Verification items for the finished model (mm, model axes). A direction names the side the tool comes from. Coordinates: 2 decimals unless noted, no trailing zeros. Loops run counter-clockwise (first coordinate to the right, second up) from the corner with the lowest first, then second, coordinate; pieces in that order, holes last. Notation, with made-up numbers: (62, 80) -> (71, 80) arc R16 ccw to (71, 89) -> close; hole circle Ø4 at (83.5, 55.5). An arc over 180 degrees is marked (long way). Write item = value, one per line.
```python
from build123d import *

# Parameters (mm, degrees)
MAINBODYS_R           = 2.5
MAIN_BODY_DEPTH       = 2
M3X0_5_TAPPED_HOLE1_D = 2.5
GROOVED_CUT_DEPTH     = 6.338539126
GC_START              = -2
GC_CP_DEPTH           = 4
PRESSFITBODYS_R       = 2
PRESSFITBODYS_R_2     = 1.25
PRESS_FIT_BODY_DEPTH  = 1


# Read off the part's stored shape, not the designer's step: GC CP
with BuildPart() as part:
    # MainBodyS → MAIN BODY (new, symmetric)
    with BuildSketch(Plane(origin=(0, 0, 0), x_dir=(1, 0, 0), z_dir=(0, 1, 0))):
        with Locations(Location((0, 0, 0), (0, 0, 270))):
            Circle(MAINBODYS_R)
    extrude(amount=MAIN_BODY_DEPTH, both=True)

    # M3x0.5 Tapped Hole1 (through all)
    with Locations(Plane(origin=(0, 2, 0), x_dir=(1, 0, 0), z_dir=(0, 1, 0))):
        with Locations((0, 0)):
            Hole(M3X0_5_TAPPED_HOLE1_D / 2)

    # GroovedCutS → GROOVED CUT (cut, through all)
    with BuildSketch(Plane(origin=(0, 2, 0), x_dir=(1, 0, 0), z_dir=(0, 1, 0))):
        with BuildLine():
            Line((0, 2.25), (0.382129822, 2.470622755))
            ThreePointArc((0.382129822, 2.470622755), (0, 2.5), (-0.382129822, 2.470622755))
            Line((-0.382129822, 2.470622755), (0, 2.25))
        make_face()
    extrude(amount=-GROOVED_CUT_DEPTH, mode=Mode.SUBTRACT)

    # GC CP outline → GC CP (cut)
    with BuildSketch(Plane(origin=(0, 0, 0), x_dir=(1, 0, 0), z_dir=(0, 1, 0)).offset(GC_START)):
        with BuildLine():
            ThreePointArc((-0.727675966, 2.391754103), (-1.084709348, 2.25242217), (-1.416250112, 2.060154271))
            Line((-1.416250112, 2.060154271), (-0.976238413, 2.027179953))
            Line((-0.976238413, 2.027179953), (-0.727675966, 2.391754103))
        make_face()
        with BuildLine():
            Line((0.976238413, 2.027179953), (1.416250112, 2.060154271))
            ThreePointArc((1.416250112, 2.060154271), (1.084709348, 2.25242217), (0.727675966, 2.391754103))
            Line((0.727675966, 2.391754103), (0.976238413, 2.027179953))
        make_face()
        with BuildLine():
            Line((1.759120836, 1.402852054), (2.169864698, 1.241646967))
            ThreePointArc((2.169864698, 1.241646967), (1.954578706, 1.558724504), (1.693356605, 1.839169217))
            Line((1.693356605, 1.839169217), (1.759120836, 1.402852054))
        make_face()
        with BuildLine():
            Line((2.193587802, 0.500672101), (2.493710969, 0.177216254))
            ThreePointArc((2.493710969, 0.177216254), (2.43731978, 0.556302335), (2.3236472, 0.922314312))
            Line((2.3236472, 0.922314312), (2.193587802, 0.500672101))
        make_face()
        with BuildLine():
            Line((2.193587802, -0.500672101), (2.3236472, -0.922314312))
            ThreePointArc((2.3236472, -0.922314312), (2.43731978, -0.556302335), (2.493710969, -0.177216254))
            Line((2.493710969, -0.177216254), (2.193587802, -0.500672101))
        make_face()
        with BuildLine():
            Line((1.759120836, -1.402852054), (1.693356605, -1.839169217))
            ThreePointArc((1.693356605, -1.839169217), (1.954578706, -1.558724504), (2.169864698, -1.241646967))
            Line((2.169864698, -1.241646967), (1.759120836, -1.402852054))
        make_face()
        with BuildLine():
            Line((0.976238413, -2.027179953), (0.727675966, -2.391754103))
            ThreePointArc((0.727675966, -2.391754103), (1.084709348, -2.25242217), (1.416250112, -2.060154271))
            Line((1.416250112, -2.060154271), (0.976238413, -2.027179953))
        make_face()
        with BuildLine():
            Line((0, -2.25), (-0.382129822, -2.470622755))
            ThreePointArc((-0.382129822, -2.470622755), (0, -2.5), (0.382129822, -2.470622755))
            Line((0.382129822, -2.470622755), (0, -2.25))
        make_face()
        with BuildLine():
            Line((-0.976238413, -2.027179953), (-1.416250112, -2.060154271))
            ThreePointArc((-1.416250112, -2.060154271), (-1.084709348, -2.25242217), (-0.727675966, -2.391754103))
            Line((-0.727675966, -2.391754103), (-0.976238413, -2.027179953))
        make_face()
        with BuildLine():
            Line((-1.759120836, -1.402852054), (-2.169864698, -1.241646967))
            ThreePointArc((-2.169864698, -1.241646967), (-1.954578706, -1.558724504), (-1.693356605, -1.839169217))
            Line((-1.693356605, -1.839169217), (-1.759120836, -1.402852054))
        make_face()
        with BuildLine():
            Line((-2.193587802, -0.500672101), (-2.493710969, -0.177216254))
            ThreePointArc((-2.493710969, -0.177216254), (-2.43731978, -0.556302335), (-2.3236472, -0.922314312))
            Line((-2.3236472, -0.922314312), (-2.193587802, -0.500672101))
        make_face()
        with BuildLine():
            Line((-2.193587802, 0.500672101), (-2.3236472, 0.922314312))
            ThreePointArc((-2.3236472, 0.922314312), (-2.43731978, 0.556302335), (-2.493710969, 0.177216254))
            Line((-2.493710969, 0.177216254), (-2.193587802, 0.500672101))
        make_face()
        with BuildLine():
            Line((-1.759120836, 1.402852054), (-1.693356605, 1.839169217))
            ThreePointArc((-1.693356605, 1.839169217), (-1.954578706, 1.558724504), (-2.169864698, 1.241646967))
            Line((-2.169864698, 1.241646967), (-1.759120836, 1.402852054))
        make_face()
    extrude(amount=GC_CP_DEPTH, mode=Mode.SUBTRACT)

    # PressFitBodyS → PRESS FIT BODY (add)
    with BuildSketch(Plane(origin=(0, 2, 0), x_dir=(1, 0, 0), z_dir=(0, 1, 0))):
        with Locations(Location((0, 0, 0), (0, 0, 270))):
            Circle(PRESSFITBODYS_R)
        with Locations(Location((0, 0, 0), (0, 0, 270))):
            Circle(PRESSFITBODYS_R_2, mode=Mode.SUBTRACT)
    extrude(amount=PRESS_FIT_BODY_DEPTH)


solid = part.part
```
1) Sectioned sample at A-A, the plane z = 0. Record the cut outline in (x, y).
Ans:
outline = (-2.5, -2) -> (-1.25, -2) -> (-1.25, 3) -> (-2, 3) -> (-2, 2) -> (-2.5, 2) -> close; (1.25, -2) -> (2.5, -2) -> (2.5, 2) -> (2, 2) -> (2, 3) -> (1.25, 3) -> close
2) Depth check by flat-ended pin: pin 1 Ø1.5 at (x, y) = (-2, -1) entering from -Z; pin 2 Ø1.5 at (x, z) = (0, 0) entering from -Y. Enter the tip coordinate at first touch or a pass-through.
Ans:
pin_1 = -2.06
pin_2 = through
3) Sectioned sample at C-C, the plane y = 2.35. Record the cut outline in (x, z), plus the area to 3 significant figures.
Ans:
outline = circle Ø4 at (0, 0); hole circle Ø2.5 at (0, 0)
area = 7.66 mm2
4) Sectioned sample at B-B, the plane x = 1.1. Record the cut outline in (y, z).
Ans:
outline = (-2, -2.04) -> (2, -2.04) -> (2, -1.67) -> (3, -1.67) -> (3, -0.59) -> (-2, -0.59) -> close; (-2, 0.59) -> (3, 0.59) -> (3, 1.67) -> (2, 1.67) -> (2, 2.04) -> (-2, 2.04) -> close
5) Sectioned sample at D-D, the plane z = -1.5. Record the cut outline in (x, y).
Ans:
outline = (-1.74, -2) -> (1.74, -2) -> (1.74, 2) -> (1.32, 2) -> (1.32, 3) -> (-1.32, 3) -> (-1.32, 2) -> (-1.74, 2) -> close
6) Material ranges on line 1 (X direction, y = 2.5, z = 0); line 2 (Y direction, x = 2.1, z = -1); line 3 (Z direction, x = 0.85, y = 2.25), recorded low to high.
Ans:
line_1 = -2 to -1.25, 1.25 to 2
line_2 = -2 to 2
line_3 = -1.81 to -0.92, 0.92 to 1.81
7) Tool access check on faces 1 (the face through (-1.952, 2.493, -0.434)), 2 (the face through (1, -2, -1)). Record the directions out of +Z, -Z, +X, -X, +Y, -Y that give a thin tool (end or side, any length) a straight path to the whole face; none if there is none.
Ans:
face_1 = +Y
face_2 = +Z, -Z, +X, -X, -Y
